from build123d import *

# Parameters (mm, degrees)
F1_DEPTH = 50.8
F3_D     = 5.5


with BuildPart() as f1:
    # F0 (on Front) → F1 (new body)
    with BuildSketch(Plane.XZ):
        with BuildLine():
            ThreePointArc((0, 6.35), (1.8598719395, 1.8598719395), (6.35, 0))
            Line((6.35, 0), (65.4343323946, 0))
            ThreePointArc((65.4343323946, 0), (69.9244604551, 1.8598719395), (71.7843323946, 6.35))
            Line((71.7843323946, 6.35), (71.7843323946, 26.8787885249))
            ThreePointArc((71.7843323946, 26.8787885249), (69.9244604551, 31.3689165854), (65.4343323946, 33.2287885249))
            Line((65.4343323946, 33.2287885249), (6.35, 33.2287885249))
            ThreePointArc((6.35, 33.2287885249), (1.8598719395, 31.3689165854), (0, 26.8787885249))
            Line((0, 26.8787885249), (0, 6.35))
        make_face()
    extrude(amount=F1_DEPTH)

    # F3 (through all)
    with Locations(Plane.XY.offset(33.2287885249)):
        with Locations((35.8921661973, -6.2919375487)):
            Hole(F3_D / 2)


solid = f1.part
Design review of the part built by this model. Coordinates are the model's own, in mm. Round coordinates to 2 decimals unless told otherwise and drop trailing zeros. Write each loop counter-clockwise with the first axis right and the second up, starting at its lowest first coordinate (ties: lowest second). Pieces come first, ordered by that corner, then holes.
Item 1: Wall thickness on L1, parallel to X at y = -6, z = 25.5; L2, parallel to X at y = -8.5, z = 21; L3, parallel to Z at x = 4, y = -39.5: over which ranges is each line inside the solid? List them lowest first.
Item 2: Consider section A-A on y = -7.5. Give the boundary of the cut face in (x, z), and give its area (3 significant figures).
Item 3: Draft analysis for pull direction Y (two halves, no side actions). For faces 1 (the cylindrical face through (38.64, -6.17, 16.38)), 2 (the flat face through (71.784, -25, 16)), 3 (the flat face through (35, -50.8, 17)), state which applies: released by +Y, released by -Y, zero draft, split by the parting line, or undercut.
Item 4: Consider section B-B on z = 3. Give the boundary of the cut face in (x, y), and give its area (3 significant figures).
Item 5: For pin 1 Ø9 at (x, y) = (35.89, -6.29) entering from -Z, flat-tipped, find the tip position at first contact; note if it passes through.
Item 6: Consider section C-C on x = 4.5. Give the boundary of the cut face in (y, z), and give its area (3 significant figures).
Check values:
1. L1: x = 0 to 33.16, 38.63 to 71.78
1. L2: x = 0 to 34.25, 37.53 to 71.78
1. L3: z = 0.45 to 32.78
2. outline: (0, 6.35) arc R6.35 ccw to (6.35, 0) - (33.42, 0) - (33.42, 33.23) - (6.35, 33.23) arc R6.35 ccw to (0, 26.88) - close; (38.36, 0) - (65.43, 0) arc R6.35 ccw to (71.78, 6.35) - (71.78, 26.88) arc R6.35 ccw to (65.43, 33.23) - (38.36, 33.23) - close
2. area: 2,190 mm2
3. face 1: undercut
3. face 2: zero draft
3. face 3: released by -Y
4. outline: (0.96, -50.8) - (70.83, -50.8) - (70.83, 0) - (0.96, 0) - close; hole circle Ø5.5 at (35.89, -6.29)
4. area: 3,530 mm2
5. pin 1: stops at z = 0
6. outline: (-50.8, 0.28) - (0, 0.28) - (0, 32.95) - (-50.8, 32.95) - close
6. area: 1,660 mm2
